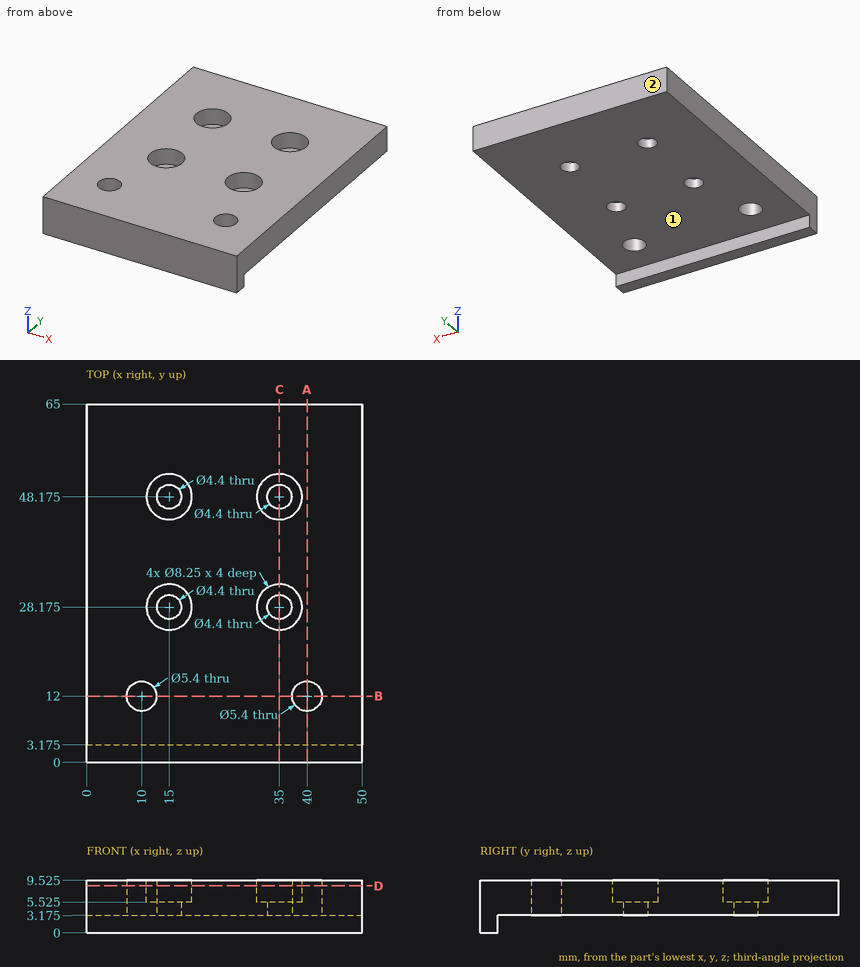
The drawing under review shows one solid part. Ordinate dimensions are in mm from its lowest x, y, z. A direction names the side the tool comes from. Coordinates: 2 decimals unless noted, no trailing zeros. Order: outer loops, then holes, each group sorted by start corner. A loop starts at its lowest first (then second) coordinate and runs counter-clockwise, first axis right, second up. Notation, with made-up numbers: (-3.75, 21) -> (27.25, 21) arc R25 ccw to (27.25, 43) -> close; hole circle Ø9 at (-5, -32.75). An arc over 180 degrees is marked (long way). Answer in a Markdown table with one row per item. Add a question column.
Item 1: Clearance check with flat-ended pins moving along their axes: pin 1 (4 mm diameter, centred on x = 15.5, y = 29, fed in from +Z) (3 decimals); pin 2 (5.5 mm diameter, centred on x = 35, y = 48.175, fed in from -Z) (3 decimals); pin 3 (1 mm diameter, centred on x = 34, z = 2, fed in from +Y) (3 decimals). State where each tip first meets the part, or that it passes through.
Item 2: Machinability: for the marked faces 1 and 2, which of the approach directions +Z, -Z, +X, -X, +Y, -Y give a long, thin tool a straight path to every point of the face, cutting with its end or side? Answer none if there is none.
Item 3: We need section D-D on z = 8.5. Write out the cut boundary in (x, y) (3 decimals).
Item 4: To check wall thickness, follow probe 1 along Y at (x, z) = (15, 8.05); probe 2 along Y at (x, z) = (35, 4.5) (3 decimals); probe 3 along Y at (x, z) = (10, 5.5). State the ranges of each line that lie inside material, in increasing order.
Item 5: We need section C-C on x = 35. Write out the cut boundary in (y, z) (3 decimals).
Item 6: We need section A-A on x = 40. Write out the cut boundary in (y, z) (3 decimals), plus the area to 3 significant figures.
Item 7: We need section B-B on y = 12. Write out the cut boundary in (x, z) (3 decimals), plus the area to 3 significant figures.
Final values:
| question | item | result |
|---|---|---|
| 1 | pin 1 | stops at z = 5.525 |
| 1 | pin 2 | stops at z = 3.175 |
| 1 | pin 3 | stops at y = 3.175 |
| 2 | face 1 | -Z, +X, -X, +Y |
| 2 | face 2 | +Z, -Z, +X, -X, +Y |
| 3 | outline | (0, 0) -> (50, 0) -> (50, 65) -> (0, 65) -> close; hole circle Ø5.4 at (10, 12); hole circle Ø8.25 at (15, 28.175); hole circle Ø8.25 at (15, 48.175); hole circle Ø8.25 at (35, 28.175); hole circle Ø8.25 at (35, 48.175); hole circle Ø5.4 at (40, 12) |
| 4 | probe 1 | y = 0 to 24.05, 32.3 to 44.05, 52.3 to 65 |
| 4 | probe 2 | y = 0 to 25.975, 30.375 to 45.975, 50.375 to 65 |
| 4 | probe 3 | y = 0 to 9.3, 14.7 to 65 |
| 5 | outline | (0, 0) -> (3.175, 0) -> (3.175, 3.175) -> (25.975, 3.175) -> (25.975, 5.525) -> (24.05, 5.525) -> (24.05, 9.525) -> (0, 9.525) -> close; (30.375, 3.175) -> (45.975, 3.175) -> (45.975, 5.525) -> (44.05, 5.525) -> (44.05, 9.525) -> (32.3, 9.525) -> (32.3, 5.525) -> (30.375, 5.525) -> close; (50.375, 3.175) -> (65, 3.175) -> (65, 9.525) -> (52.3, 9.525) -> (52.3, 5.525) -> (50.375, 5.525) -> close |
| 6 | outline | (0, 0) -> (3.175, 0) -> (3.175, 3.175) -> (9.3, 3.175) -> (9.3, 9.525) -> (0, 9.525) -> close; (14.7, 3.175) -> (65, 3.175) -> (65, 9.525) -> (14.7, 9.525) -> close |
| 6 | area | 389 mm2 |
| 7 | outline | (0, 3.175) -> (7.3, 3.175) -> (7.3, 9.525) -> (0, 9.525) -> close; (12.7, 3.175) -> (37.3, 3.175) -> (37.3, 9.525) -> (12.7, 9.525) -> close; (42.7, 3.175) -> (50, 3.175) -> (50, 9.525) -> (42.7, 9.525) -> close |
| 7 | area | 249 mm2 |
